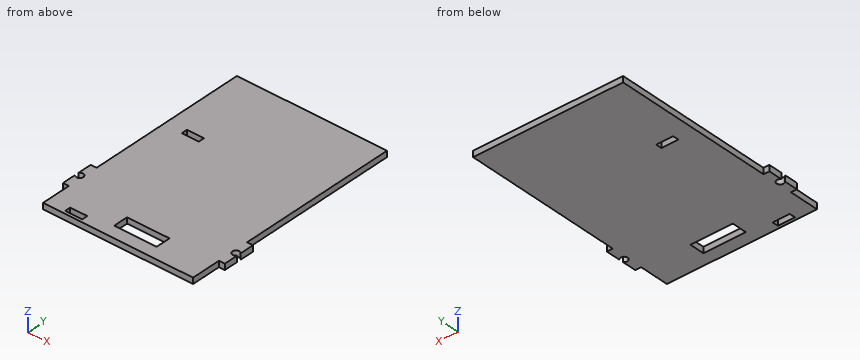
```python
from build123d import *

# Parameters (mm, degrees)
SKETCH1_W           = 87
SKETCH1_H           = 44.45
SKETCH1_W_2         = 9.142679105
SKETCH1_H_2         = 3.175
BOSS_EXTRUDE1_DEPTH = 3.175
SKETCH2_W           = 3.175
SKETCH2_H           = 11.14
CUT_EXTRUDE1_DEPTH  = 4.175
SKETCH3_W           = 3.175
SKETCH3_H           = 15.88
CUT_EXTRUDE2_DEPTH  = 4.175
SKETCH6_R           = 1.905
CUT_EXTRUDE3_DEPTH  = 4.175
SKETCH8_W           = 3.175
SKETCH8_H           = 11.469011162
SKETCH8_H_2         = 15.983017012
CUT_EXTRUDE4_DEPTH  = 4.175
SKETCH10_R          = 1.905
CUT_EXTRUDE5_DEPTH  = 4.175
SKETCH12_W          = 80.65
SKETCH12_H          = 3.175
BOSS_EXTRUDE2_DEPTH = 75
SKETCH18_W          = 9.14
SKETCH18_H          = 3.18
CUT_EXTRUDE6_DEPTH  = 3.18
SKETCH19_W          = 22.786874906
SKETCH19_H          = 7.908464624
CUT_EXTRUDE7_DEPTH  = 3.18


with BuildPart() as part:
    # Sketch1 → Boss-Extrude1 (new body)
    with BuildSketch(Plane.XY):
        with Locations((43.5, -22.225)):
            Rectangle(SKETCH1_W, SKETCH1_H)
        with Locations((18.232073224, -41.2725)):
            Rectangle(SKETCH1_W_2, SKETCH1_H_2, mode=Mode.SUBTRACT)
    extrude(amount=BOSS_EXTRUDE1_DEPTH)

    # Sketch2 → Cut-Extrude1 (cut, through all)
    with BuildSketch(Plane(origin=(0, 0, 0), x_dir=(-1, 0, 0), z_dir=(0, 0, -1))):
        with Locations((-85.4125, -5.57)):
            Rectangle(SKETCH2_W, SKETCH2_H)
    extrude(amount=-CUT_EXTRUDE1_DEPTH, mode=Mode.SUBTRACT)

    # Sketch3 → Cut-Extrude2 (cut, through all)
    with BuildSketch(Plane(origin=(0, 0, 0), x_dir=(-1, 0, 0), z_dir=(0, 0, -1))):
        with Locations((-85.4125, -36.51)):
            Rectangle(SKETCH3_W, SKETCH3_H)
    extrude(amount=-CUT_EXTRUDE2_DEPTH, mode=Mode.SUBTRACT)

    # Sketch6 → Cut-Extrude3 (cut, through all)
    with BuildSketch(Plane(origin=(0, 0, 0), x_dir=(-1, 0, 0), z_dir=(0, 0, -1))):
        with Locations((-85.4125, -19.855)):
            Circle(SKETCH6_R)
    extrude(amount=-CUT_EXTRUDE3_DEPTH, mode=Mode.SUBTRACT)

    # Sketch8 → Cut-Extrude4 (cut, through all)
    with BuildSketch(Plane(origin=(0, 0, 0), x_dir=(-1, 0, 0), z_dir=(0, 0, -1))):
        with Locations((-1.5875, -5.734505581)):
            Rectangle(SKETCH8_W, SKETCH8_H)
        with Locations((-1.5875, -36.458491494)):
            Rectangle(SKETCH8_W, SKETCH8_H_2)
    extrude(amount=-CUT_EXTRUDE4_DEPTH, mode=Mode.SUBTRACT)

    # Sketch10 → Cut-Extrude5 (cut, through all)
    with BuildSketch(Plane(origin=(0, 0, 0), x_dir=(-1, 0, 0), z_dir=(0, 0, -1))):
        with Locations((-1.5875, -19.967997075)):
            Circle(SKETCH10_R)
    extrude(amount=-CUT_EXTRUDE5_DEPTH, mode=Mode.SUBTRACT)

    # Sketch12 → Boss-Extrude2 (add)
    with BuildSketch(Plane(origin=(0, 0, 0), x_dir=(1, 0, 0), z_dir=(0, 1, 0))):
        with Locations((43.5, -1.5875)):
            Rectangle(SKETCH12_W, SKETCH12_H)
    extrude(amount=BOSS_EXTRUDE2_DEPTH)

    # Sketch18 → Cut-Extrude6 (cut)
    with BuildSketch(Plane.XY.offset(3.175)):
        with Locations((17.561709366, 31.346582601)):
            Rectangle(SKETCH18_W, SKETCH18_H)
    extrude(amount=-CUT_EXTRUDE6_DEPTH, mode=Mode.SUBTRACT)

    # Sketch19 → Cut-Extrude7 (cut)
    with BuildSketch(Plane.XY.offset(3.175)):
        with Locations((46.923268397, -33.695818912)):
            Rectangle(SKETCH19_W, SKETCH19_H)
    extrude(amount=-CUT_EXTRUDE7_DEPTH, mode=Mode.SUBTRACT)


solid = part.part
```
Could you check a few things on this model? Use its own coordinates, in mm. Coordinates: 2 decimals unless noted, no trailing zeros. Loops run counter-clockwise (first coordinate to the right, second up) from the corner with the lowest first, then second, coordinate; pieces in that order, holes last.
1) Will these pins go through, and if not, where does the flat tip stop? pin 1 Ø3.5 at (x, y) = (85.41, -19.86) entering from +Z; pin 2 Ø1.5 at (y, z) = (8.5, 2) entering from +X (3 decimals); pin 3 Ø1.6 at (y, z) = (-41, 1) entering from -X (3 decimals); pin 4 Ø1 at (x, z) = (84.5, 2) entering from +Y.
Reported:
pin 1: passes through
pin 2: stops at x = 83.825
pin 3: stops at x = 3.175
pin 4: stops at y = -11.14
2) Imagine slicing it at C-C (y = -34). List the corners of the cut face in (x, z) for me (3 decimals).
Reported:
outline: (3.175, 0) - (35.53, 0) - (35.53, 3.175) - (3.175, 3.175) - close; (58.317, 0) - (83.825, 0) - (83.825, 3.175) - (58.317, 3.175) - close
3) Imagine slicing it at A-A (x = 19.5). List the corners of the cut face in (y, z) for me (3 decimals), and give its area (3 significant figures).
Reported:
outline: (-44.45, 0) - (-42.86, 0) - (-42.86, 3.175) - (-44.45, 3.175) - close; (-39.685, 0) - (29.757, 0) - (29.757, 3.175) - (-39.685, 3.175) - close; (32.937, 0) - (75, 0) - (75, 3.175) - (32.937, 3.175) - close
area: 359 mm2
4) Imagine slicing it at B-B (x = 50). List the corners of the cut face in (y, z) for me (3 decimals), and give its area (3 significant figures).
Reported:
outline: (-44.45, 0) - (-37.65, 0) - (-37.65, 3.175) - (-44.45, 3.175) - close; (-29.742, 0) - (75, 0) - (75, 3.175) - (-29.742, 3.175) - close
area: 354 mm2
5) Imagine slicing it at D-D (z = 1.75). State how many separate pieces and enclosed holes the cut face has, and give its area (3 significant figures).
Reported:
separate pieces: 1
enclosed holes: 3
area: 9,480 mm2
6) Please list where these lines run through material, in increasing order: line 1 along Y through (x, z) = (15.5, 1.85) (3 decimals); line 2 along X through (y, z) = (-32.5, 0.1) (3 decimals); line 3 along Y through (x, z) = (44, 2.9).
Reported:
line 1: y = -44.45 to -42.86, -39.685 to 29.757, 32.937 to 75
line 2: x = 3.175 to 35.53, 58.317 to 83.825
line 3: y = -44.45 to -37.65, -29.74 to 75
